```python
from build123d import *

# Parameters (mm, degrees)
ESBO_O1_W                = 150
ESBO_O1_H                = 20
RESSALTO_EXTRUS_O1_DEPTH = 490
CHANFRO1_SIZE            = 20
ESBO_O2_R                = 25
CORTE_EXTRUS_O1_DEPTH    = 513.835256198
CHANFRO2_SIZE2           = 20
CHANFRO2_SIZE            = 8.284271247


# Some blends are built 0.0001 mm under size
with BuildPart() as part:
    # Esboço1 → Ressalto-extrusão1 (new body)
    with BuildSketch(Plane.XY):
        with Locations((75, 10)):
            Rectangle(ESBO_O1_W, ESBO_O1_H)
    extrude(amount=RESSALTO_EXTRUS_O1_DEPTH)

    # Chanfro1
    # the kernel refuses this chamfer: 20 mm, written as the material it takes off along each edge
    with BuildSketch(Plane(origin=(-51.433659759, 0, 490), x_dir=(0, -0.027495876610586334, -0.9996219169112968), z_dir=(1, 0, 0))) as chanfro1_piece_1:
        Polygon((CHANFRO1_SIZE * 0.999621916911, CHANFRO1_SIZE * 0.0274958766106), (-CHANFRO1_SIZE * 0.0274958766106, CHANFRO1_SIZE * 0.999621916911), (0, 0), align=None)
    extrude(amount=252.867319519, mode=Mode.SUBTRACT)
    with BuildSketch(Plane(origin=(0, 0, -51.433659759), x_dir=(0.9996219169112968, -0.027495876610586372, 0), z_dir=(0, 0, 1))) as chanfro1_piece_2:
        Polygon((CHANFRO1_SIZE * 0.999621916911, CHANFRO1_SIZE * 0.0274958766106), (-CHANFRO1_SIZE * 0.0274958766106, CHANFRO1_SIZE * 0.999621916911), (0, 0), align=None)
    extrude(amount=592.867319519, mode=Mode.SUBTRACT)
    with BuildSketch(Plane(origin=(-51.433659759, 0, 0), x_dir=(0, -0.027495876610586372, 0.9996219169112968), z_dir=(1, 0, 0))) as chanfro1_piece_3:
        Polygon((CHANFRO1_SIZE * 0.999621916911, -CHANFRO1_SIZE * 0.0274958766106), (-CHANFRO1_SIZE * 0.0274958766106, -CHANFRO1_SIZE * 0.999621916911), (0, 0), align=None)
    extrude(amount=252.867319519, mode=Mode.SUBTRACT)

    # Esboço2 → Corte-extrusão1 (cut, through all)
    with BuildSketch(Plane(origin=(0, 0, 0), x_dir=(-1, 0, 0), z_dir=(0, -1, 0))):
        with Locations(Location((-75, -245, 0), (0, 0, 90))):
            Circle(ESBO_O2_R)
    extrude(amount=-CORTE_EXTRUS_O1_DEPTH, mode=Mode.SUBTRACT)

    # Chanfro2
    chanfro2_edges = [part.edges().sort_by_distance(p)[0] for p in [
        (150, 0, 245),
    ]]
    chanfro2_side = [part.faces().sort_by_distance(p)[0] for p in [
        (149.834314575, 0, 245),
    ]]
    chamfer(chanfro2_edges, length=CHANFRO2_SIZE - 0.0001, length2=CHANFRO2_SIZE2 - 0.0001, reference=chanfro2_side[0])  # a hair under: the kernel refuses the full size


solid = part.part
```
Input: part model. Units: mm. Frame: model coordinates. Give positions to 0.01 mm unless a question says otherwise; leave off trailing zeros. Order: outer loops, then holes, each group sorted by start corner. A loop starts at its lowest first (then second) coordinate and runs counter-clockwise, first axis right, second up. Notation, with made-up numbers: (7, 84.5) - (25, 84.5) arc R5 ccw to (25, 92.5) - close; hole circle Ø8 at (34.25, 29). An arc over 180 degrees is marked (long way). Put each result on its own line as item: value.
Item 1: Ray query, L1, parallel to Z at x = 56, y = 18.75; L2, parallel to X at y = 15, z = 245; L3, parallel to X at y = 9.25, z = 245. Return the intervals inside material, ascending. Write a range as from..to.
Found:
L1: z = 1.25..228.75, 261.25..488.75
L2: x = 5..50, 100..147.93
L3: x = 10.75..50, 100..145.55
Item 2: Section query C-C, the plane y = 15.5. Return loops of the section in (x, z), then the cut area to 3 significant figures.
Found:
outline: (4.5, 4.5) - (148.14, 4.5) - (148.14, 485.5) - (4.5, 485.5) - close; hole circle Ø50 at (75, 245)
area: 67,100 mm^2
Item 3: Section query A-A, the plane x = 75. Return loops of the section in (y, z).
Found:
outline: (0, 20) - (20, 0) - (20, 220) - (0, 220) - close; (0, 270) - (20, 270) - (20, 490) - (0, 470) - close
Item 4: Contact query for flat-ended pins moving along their axis: pin 1 (1.5 mm diameter, centred on x = 110, y = 13, fed in from +Z); pin 2 (1.5 mm diameter, centred on y = 14.5, z = 288, fed in from -X); pin 3 (3 mm diameter, centred on x = 65, y = 7, fed in from +Z). Output: stop coordinate, or through.
Found:
pin 1: stops at z = 483.75
pin 2: stops at x = 4.75
pin 3: stops at z = 478.5
Item 5: Draft query along Z for faces 1 (the flat face through (10, 10, 242)), 2 (the cylindrical face through (65.42, 9.86, 221.91)), 3 (the flat face through (74, 10, 10)), 4 (the flat face through (74, 10, 480)). Return one class per face: +Z half, -Z half, draft (parallel to the pull), parting line (faces both ways), or undercut.
Found:
face 1: draft
face 2: undercut
face 3: -Z half
face 4: +Z half
